Autodesk Inventor part; units mm, degrees
ref_plane "YZ Plane" through (0, 0, 0) normal (1, 0, 0) x (0, 1, 0)
ref_plane "XZ Plane" through (0, 0, 0) normal (0, 1, 0) x (-1, 0, 0)
ref_plane "XY Plane" through (0, 0, 0) normal (0, 0, 1) x (1, 0, 0)
sketch "Sketch1" plane through (0, 0, 0) normal (0, 1, 0) x (-1, 0, 0)
  line L0 (0, 0) -> (0, -46.0375)
  line L1 (0, 0) -> (20.32, 0)
  line L2 (16.6421, -3.175) -> (0, -3.175)
  line L3 (0, -3.175) -> (0, 0)
  line L4 (0, -46.0375) -> (57.15, -46.0375)
  line L5 (0, -46.0375) -> (57.15, -46.0375) construction
  line L6 (20.32, 0) -> (59.69, 0) construction
  line L7 (20.32, -3.175) -> (52.07, -3.175) construction
  arc A0 (75.1105, -28.077) -> (57.15, -46.0375) centre (75.1105, -46.0375) ccw
  line L8 (57.15, -46.0375) -> (75.1105, -28.077) construction
  line L9 (57.15, -46.0375) -> (82.55, -46.0375) construction
  line L10 (20.32, 0) -> (58.8119, -38.4919)
  line L11 (20.32, 0) -> (74.7558, 0) construction
  line L12 (20.32, -3.175) -> (72.6455, -3.175) construction
  line L13 (0, -92.075) -> (0, -46.0375)
  line L14 (16.6421, -3.175) -> (46.6548, -46.0375)
  line L15 (16.6421, -3.175) -> (68.9676, -3.175) construction
  line L16 (0, -92.075) -> (0, -46.0375)
  line L17 (0, -92.075) -> (20.32, -92.075)
  line L18 (16.6421, -88.9) -> (0, -88.9)
  line L19 (0, -88.9) -> (0, -92.075)
  line L20 (20.32, -92.075) -> (59.69, -92.075) construction
  line L21 (20.32, -88.9) -> (52.07, -88.9) construction
  arc A1 (57.15, -46.0375) -> (75.1105, -63.998) centre (75.1105, -46.0375) ccw
  line L22 (57.15, -46.0375) -> (75.1105, -63.998) construction
  line L23 (20.32, -92.075) -> (58.8119, -53.5831)
  line L24 (20.32, -92.075) -> (74.7558, -92.075) construction
  line L25 (20.32, -88.9) -> (72.6455, -88.9) construction
  line L26 (16.6421, -88.9) -> (46.6548, -46.0375)
  line L27 (16.6421, -88.9) -> (68.9676, -88.9) construction
  dimension "d1" = 20.32
  dimension "d6" = 0
  dimension "d26" = 25.4
  dimension "d27" = 45
  dimension "d29" = 45
  dimension "d31" = 55
  dimension "d34" = 92.075
extrude "Extrusion1" add sketch "Sketch1" along normal blind 25.4 contours L1 L10 A0 L4 L14 L2 L0 | L4 A1 L23 L17 L13 L18 L26
sketch "Sketch2" plane through (-20.32, 0, 0) normal (0, 0, 1) x (1, 0, 0)
  line L0 (20.32, 0) -> (20.32, 25.4)
  line L1 (20.32, 12.7) -> (10.16, 12.7)
  circle A0 centre (10.16, 12.7) radius 2.54
  dimension "d19" = 10.16
  dimension "d20" = 5.08
extrude "Extrusion2" cut sketch "Sketch2" against normal blind 142.875
properties part number "NeckRest"
Geometry check sheet. Reference: the model listing, model coordinates, mm. A direction names the side the tool comes from. Round coordinates to 2 decimals unless told otherwise and drop trailing zeros. Order: outer loops, then holes, each group sorted by start corner. A loop starts at its lowest first (then second) coordinate and runs counter-clockwise, first axis right, second up. Notation, with made-up numbers: M -13.75,74 L 20.25,74 A34 cw 20.25,113 Z; hole C 67,-0.75 d7. An arc over 180 degrees is marked long. Write each question's results on one line, items separated by ' | '. Start each with the question number.
1. Set-up check for faces 1 (the face through (-31.44, 12.52, -24.31)), 2 (the face through (-7.737, 13.463, -90.465)): record each of +Z, -Z, +X, -X, +Y, -Y from which the full face is reachable in a straight line by a thin tool's end or side.
2. Go/stop test with flat-tipped pins: P1, Ø6, axis at x = -36.5, y = 5.5, coming from the +Z side; P2, Ø8, axis at x = -30.5, y = 10.5, coming from the +Z side; P3, Ø2, axis at x = -14, y = 18.5, coming from the +Z side; P4, Ø2, axis at y = 20, z = -27.5, coming from the -X side. Record where each tip stops, or that it passes through.
3. Material ranges on L1, parallel to Z at x = -4, y = 6.5 (3 decimals); L2, parallel to Y at x = -10.16, z = -89.9; L3, parallel to Z at x = -37, y = 20.25 (3 decimals), recorded low to high. Write a range as from..to.
4. Cross-section at B-B on y = 12.7. Record the boundary of the cut face in (x, z) (1 decimal), plus the area to 3 significant figures.
5. Cross-section at C-C on x = -22. Record the boundary of the cut face in (y, z) (3 decimals), plus the area to 3 significant figures.
6. Cross-section at D-D on y = 18.75. Record the boundary of the cut face in (x, z) (1 decimal), plus the area to 3 significant figures.
7. Draft check along Z on faces 3 (the face through (-57.15, 12.52, -46.15)), 4 (the face through (0, 13, -91)), 5 (the face through (-10, 10, 0)). Enter one of: pulls with the +Z half, pulls with the -Z half, needs draft (parallel to the pull), parting line crosses it, or undercut.
8. Cross-section at A-A on x = -14.5. Record the boundary of the cut face in (y, z) (3 decimals).
Resolved:
1) face 1: +X, +Y, -Y | face 2: +Z, -Z
2) P1: z = -13.18 | P2: z = -6.18 | P3: z = 0 | P4: x = -48.82
3) L1: -92.075..-88.9, -3.175..0 | L2: 0..10.16, 15.24..25.4 | L3: -75.395..-59.826, -32.249..-16.68
4) outline: M -58.8,-53.6 L -20.3,-92.1 L -12.7,-92.1 L -12.7,-88.9 L -16.6,-88.9 L -46.7,-46 L -16.6,-3.2 L -12.7,-3.2 L -12.7,0 L -20.3,0 L -58.8,-38.5 A18 cw Z; M -7.6,-92.1 L 0,-92.1 L 0,-88.9 L -7.6,-88.9 Z; M -7.6,-3.2 L 0,-3.2 L 0,0 L -7.6,0 Z | area: 1,170 mm2
5) outline: M 0,-90.395 L 25.4,-90.395 L 25.4,-81.248 L 0,-81.248 Z; M 0,-10.827 L 25.4,-10.827 L 25.4,-1.68 L 0,-1.68 Z | area: 465 mm2
6) outline: M -58.8,-53.6 L -20.3,-92.1 L 0,-92.1 L 0,-88.9 L -16.6,-88.9 L -46.7,-46 L -16.6,-3.2 L 0,-3.2 L 0,0 L -20.3,0 L -58.8,-38.5 A18 cw Z | area: 1,200 mm2
7) face 3: undercut | face 4: needs draft | face 5: pulls with the +Z half
8) outline: M 0,-92.075 L 25.4,-92.075 L 25.4,-88.9 L 0,-88.9 Z; M 0,-3.175 L 25.4,-3.175 L 25.4,0 L 0,0 Z
